Source: CAD feature listing. Evaluate the final solid. Frame: model axes, mm. Face numbers are marked on the shaded views. A direction names the side the tool comes from. Coordinates: 2 decimals unless noted, no trailing zeros. Order: outer loops, then holes, each group sorted by start corner. A loop starts at its lowest first (then second) coordinate and runs counter-clockwise, first axis right, second up. Notation, with made-up numbers: (56, 87) - (81, 87) arc R33 ccw to (81, 123) - close; hole circle Ø7 at (60.25, 84). An arc over 180 degrees is marked (long way). One line per question, with ' | ' between items. Start each with the question number.
(1) Line query: line 1 along Y through (x, z) = (0, 0.15); line 2 along Y through (x, z) = (17.5, 1.05); line 3 along X through (y, z) = (14, -1.7). Output: solid intervals per line, ascending.
(2) Contact query for flat-ended pins moving along their axis: P1, Ø2.5, axis at x = -24.27, y = -14.61, coming from the +Z side; P2, Ø2, axis at y = 7, z = -0.5, coming from the -X side; P3, Ø0.5, axis at x = 10.5, z = -0.5, coming from the -Y side; P4, Ø1.5, axis at x = -12, z = -0.5, coming from the +Y side. Output: stop coordinate, or through.
(3) Section B-B (y = -2.5). Count the separate pieces of the cut face and the enclosed holes in it, then the cut area to 3 significant figures.
(4) Access query for the marked faces 4, 5 and 6. Directions: +Z, -Z, +X, -X, +Y, -Y. A direction counts if a zero-diameter tool reaches every point of the face in a straight line with its end or side. Return the directions, or none.
(5) Draft query along X for the marked faces 1, 2 and 3. Return one class per face: +X half, -X half, draft (parallel to the pull), parting line (faces both ways), or undercut.
(6) Section A-A (x = 0). Return the cut outline in (y, z).
from build123d import *

# Parameters (mm, degrees)
SKETCH_1_R             = 7
SKETCH_1_R_2           = 1.55
EXTRUDE_1_DEPTH        = 2
FILLET_1_R             = 1
CUT_EXTRUDE_START      = -5
CUT_EXTRUDE_1_DEPTH    = 6
FILLET_2_R             = 1
FILLET_2_OF_MIRROR_1_R = 1
SKETCH_3_R             = 1.55
EXTRUDE_2_DEPTH        = 4
FILLET_3_R             = 1
CUT_EXTRUDE_2_DEPTH    = 5
FILLET_4_R             = 1
CUT_EXTRUDE_3_DEPTH    = 5
EXTRUDE_3_DEPTH        = 4
SKETCH_8_R             = 0.75
CUT_EXTRUDE_4_DEPTH    = 5
FILLET_5_R             = 1.5


with BuildPart() as part:
    # 草图1 → 凸台-拉伸1 (new body, symmetric)
    with BuildSketch(Plane.XY):
        with BuildLine():
            Line((-17.5, 11), (-10, 11))
            Line((-10, 11), (-8.321800738, 9))
            Line((-8.321800738, 9), (8.321800738, 9))
            Line((8.321800738, 9), (10, 11))
            Line((10, 11), (17.5, 11))
            ThreePointArc((17.5, 11), (17.577641076, 10.999138732), (17.655243941, 10.99655535))
            Line((17.655243941, 10.99655535), (37, 10.137665421))
            Line((37, 10.137665421), (28.942548731, -12))
            Line((28.942548731, -12), (17.199216279, -10.987051642))
            ThreePointArc((17.199216279, -10.987051642), (15.184578245, -10.124656567), (14.077678472, -8.233290774))
            Line((14.077678472, -8.233290774), (2.304628146, -10.75586766))
            ThreePointArc((2.304628146, -10.75586766), (0, -11), (-2.304628146, -10.75586766))
            Line((-2.304628146, -10.75586766), (-14.077678472, -8.233290774))
            ThreePointArc((-14.077678472, -8.233290774), (-15.184578245, -10.124656567), (-17.199216279, -10.987051642))
            Line((-17.199216279, -10.987051642), (-28.942548731, -12))
            Line((-28.942548731, -12), (-37, 10.137665421))
            Line((-37, 10.137665421), (-17.655243941, 10.99655535))
            ThreePointArc((-17.655243941, 10.99655535), (-17.577641076, 10.999138732), (-17.5, 11))
        make_face()
        Circle(SKETCH_1_R, mode=Mode.SUBTRACT)
        with Locations((17.5, 7.5)):
            Circle(SKETCH_1_R_2, mode=Mode.SUBTRACT)
        with Locations((17.5, -7.5)):
            Circle(SKETCH_1_R_2, mode=Mode.SUBTRACT)
        with Locations((-17.5, -7.5)):
            Circle(SKETCH_1_R_2, mode=Mode.SUBTRACT)
        with Locations((-17.5, 7.5)):
            Circle(SKETCH_1_R_2, mode=Mode.SUBTRACT)
    extrude(amount=EXTRUDE_1_DEPTH, both=True)

    # 圆角1
    fillet_1_edges = [part.edges().sort_by_distance(p)[0] for p in [
        (14.077678472, -8.233290774, 0),
        (-14.077678472, -8.233290774, 0),
    ]]
    fillet(fillet_1_edges, radius=FILLET_1_R)

    # 草图2 → 切除-拉伸1 (cut)
    with BuildSketch(Plane.XY.offset(2).offset(CUT_EXTRUDE_START)):
        Polygon((-20.5, 7.867295251), (-32.782632739, 7.321957304), (-27.222903771, -7.953272497), align=None)
        with BuildLine():
            Line((-19.251811465, 4.412338006), (-24.573190843, -8.11011447))
            Line((-24.573190843, -8.11011447), (-21.036866665, -7.805080632))
            ThreePointArc((-21.036866665, -7.805080632), (-20.623106229, -5.812188553), (-19.182687898, -4.374130291))
            Line((-19.182687898, -4.374130291), (-15.331076504, 4.689613751))
            ThreePointArc((-15.331076504, 4.689613751), (-17.24956823, 3.958844267), (-19.251811465, 4.412338006))
        make_face()
    cut_extrude_1 = extrude(amount=CUT_EXTRUDE_1_DEPTH, mode=Mode.SUBTRACT)

    # 圆角2
    fillet_2_edges = [part.edges().sort_by_distance(p)[0] for p in [
        (-20.5, 7.867295251, 0),
        (-27.222903771, -7.953272497, 0),
        (-32.782632739, 7.321957304, 0),
        (-19.251811465, 4.412338006, 0),
        (-15.331076504, 4.689613751, 0),
        (-19.182687898, -4.374130291, 0),
        (-21.036866665, -7.805080632, 0),
        (-24.573190843, -8.11011447, 0),
    ]]
    fillet(fillet_2_edges, radius=FILLET_2_R)

    # 镜向1: 切除-拉伸1 across plane
    add(cut_extrude_1.mirror(Plane(origin=(0, 0, 0), x_dir=(0, 0, 1), z_dir=(1, 0, 0))), mode=Mode.SUBTRACT)

    # 圆角2 of 镜向1
    fillet_2_of_mirror_1_edges = [part.edges().sort_by_distance(p)[0] for p in [
        (20.5, 7.867295251, 0),
        (27.222903771, -7.953272497, 0),
        (32.782632739, 7.321957304, 0),
        (19.251811465, 4.412338006, 0),
        (15.331076504, 4.689613751, 0),
        (19.182687898, -4.374130291, 0),
        (21.036866665, -7.805080632, 0),
        (24.573190843, -8.11011447, 0),
    ]]
    fillet(fillet_2_of_mirror_1_edges, radius=FILLET_2_OF_MIRROR_1_R)

    # 草图3 → 凸台-拉伸2 (add)
    with BuildSketch(Plane.XY.offset(2)):
        with BuildLine():
            Line((-37.69913918, 12.058534531), (-37, 10.137665421))
            Line((-37, 10.137665421), (-32.4761474, 10.338520445))
            ThreePointArc((-32.4761474, 10.338520445), (-33.315445081, 16.579981486), (-37.69913918, 12.058534531))
        make_face()
        with Locations((-34.410215007, 13.255605032)):
            Circle(SKETCH_3_R, mode=Mode.SUBTRACT)
        with BuildLine():
            Line((-27.557621455, -15.805056417), (-28.942548731, -12))
            Line((-28.942548731, -12), (-22.730405687, -11.464157204))
            ThreePointArc((-22.730405687, -11.464157204), (-21.928391725, -17.210478932), (-27.557621455, -15.805056417))
        make_face()
        with Locations((-24.268697282, -14.607985915)):
            Circle(SKETCH_3_R, mode=Mode.SUBTRACT)
    extrude_2 = extrude(amount=-EXTRUDE_2_DEPTH)

    # 镜向2: 凸台-拉伸2 across plane
    add(extrude_2.mirror(Plane(origin=(0, 0, 0), x_dir=(0, 0, 1), z_dir=(1, 0, 0))))

    # 圆角3
    fillet_3_edges = [part.edges().sort_by_distance(p)[0] for p in [
        (-22.730405687, -11.464157204, 0),
        (-32.4761474, 10.338520445, 0),
        (22.730405687, -11.464157204, 0),
        (32.4761474, 10.338520445, 0),
    ]]
    fillet(fillet_3_edges, radius=FILLET_3_R)

    # 草图4 → 切除-拉伸2 (cut, through all)
    with BuildSketch(Plane.XY.offset(2)):
        with BuildLine():
            Line((-16.384851826, -4.1824038), (-12.057869255, 6))
            Line((-12.057869255, 6), (-8, 6))
            ThreePointArc((-8, 6), (-9.993390733, -0.363512948), (-7.542930102, -6.565379309))
            Line((-7.542930102, -6.565379309), (-15.108699944, -4.944284045))
            ThreePointArc((-15.108699944, -4.944284045), (-15.705867849, -4.49482283), (-16.384851826, -4.1824038))
        make_face()
    cut_extrude_2 = extrude(amount=-CUT_EXTRUDE_2_DEPTH, mode=Mode.SUBTRACT)

    # 镜向3: 切除-拉伸2 across plane
    add(cut_extrude_2.mirror(Plane(origin=(0, 0, 0), x_dir=(0, 0, 1), z_dir=(1, 0, 0))), mode=Mode.SUBTRACT)

    # 圆角4
    fillet_4_edges = [part.edges().sort_by_distance(p)[0] for p in [
        (-12.057869255, 6, 0),
        (-8, 6, 0),
        (-7.542930102, -6.565379309, 0),
        (-15.108699944, -4.944284045, 0),
        (-16.384851826, -4.1824038, 0),
        (8, 6, 0),
        (12.057869255, 6, 0),
        (16.384851826, -4.1824038, 0),
        (15.108699944, -4.944284045, 0),
        (7.542930102, -6.565379309, 0),
    ]]
    fillet(fillet_4_edges, radius=FILLET_4_R)

    # 草图5 → 切除-拉伸3 (cut, through all)
    with BuildSketch(Plane.XY.offset(2)):
        Polygon((30.884976598, -6.370842854), (33.798023723, -7.431105298), (37.25242717, 2.059790172), (34.339380046, 3.120052616), align=None)
    cut_extrude_3 = extrude(amount=-CUT_EXTRUDE_3_DEPTH, mode=Mode.SUBTRACT)

    # 草图7 → 凸台-拉伸3 (add)
    with BuildSketch(Plane.XY.offset(2)):
        Polygon((35.271298659, 5.388097522), (40.439608074, 3.506986734), (35.309305924, -10.588402578), (30.140996509, -8.707291789), (30.97894586, -6.405044868), (33.798023723, -7.431105298), (37.25242717, 2.059790172), (34.433349308, 3.085850601), align=None)
    extrude_3 = extrude(amount=-EXTRUDE_3_DEPTH)

    # 镜向4: 切除-拉伸3, 凸台-拉伸3 across plane
    add(cut_extrude_3.mirror(Plane(origin=(0, 0, 0), x_dir=(0, 0, 1), z_dir=(1, 0, 0))), mode=Mode.SUBTRACT)
    add(extrude_3.mirror(Plane(origin=(0, 0, 0), x_dir=(0, 0, 1), z_dir=(1, 0, 0))))

    # 草图8 → 切除-拉伸4 (cut, through all)
    with BuildSketch(Plane(origin=(0, 0, -2), x_dir=(-1, 0, 0), z_dir=(0, 0, -1))):
        with Locations((-36.995912063, 1.355020706)):
            Circle(SKETCH_8_R)
        with Locations((-34.082864939, 2.41528315)):
            Circle(SKETCH_8_R)
        with Locations((-34.05453883, -6.726335833)):
            Circle(SKETCH_8_R)
        with Locations((-31.141491706, -5.666073389)):
            Circle(SKETCH_8_R)
        with Locations((-35.527813767, 6.092866988)):
            Circle(SKETCH_8_R)
        with Locations((-29.884481402, -9.412061255)):
            Circle(SKETCH_8_R)
    cut_extrude_4 = extrude(amount=-CUT_EXTRUDE_4_DEPTH, mode=Mode.SUBTRACT)

    # 镜向5: 切除-拉伸4 across plane
    add(cut_extrude_4.mirror(Plane(origin=(0, 0, 0), x_dir=(0, 0, 1), z_dir=(1, 0, 0))), mode=Mode.SUBTRACT)

    # 圆角5
    fillet_5_edges = [part.edges().sort_by_distance(p)[0] for p in [
        (40.439608074, 3.506986734, 0),
        (35.309305924, -10.588402578, 0),
        (-40.439608074, 3.506986734, 0),
        (-35.309305924, -10.588402578, 0),
    ]]
    fillet(fillet_5_edges, radius=FILLET_5_R)


solid = part.part
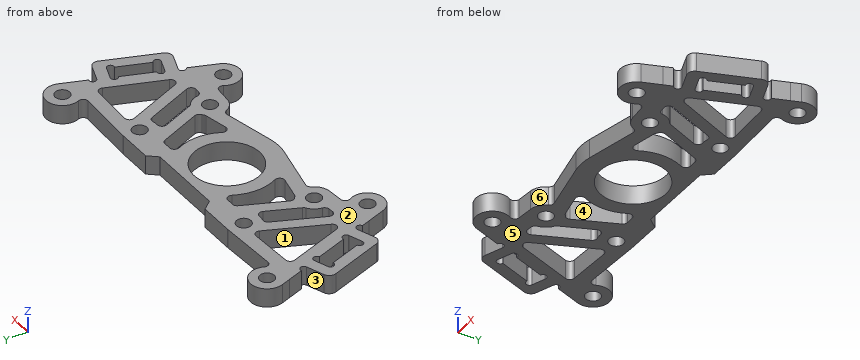
Response values:
1) line 1: y = -11 to -7, 7 to 9 | line 2: y = -11.01 to -9.05, -5.95 to -0.41, 3.95 to 5.95, 9.05 to 11 | line 3: x = -37.83 to -35.77, -33.05 to -30.99, 30.99 to 33.05, 35.77 to 37.83
2) P1: passes through | P2: stops at x = -36.22 | P3: stops at y = -9.05 | P4: stops at y = 11
3) separate pieces: 10 | enclosed holes: 0 | area: 115 mm²
4) face 4: +Z, -Z | face 5: -Z, +X, -X, +Y, -Y | face 6: +Z, -Z, -Y
5) face 1: undercut | face 2: draft | face 3: -X half
6) outline: (-11, -2) - (-7, -2) - (-7, 2) - (-11, 2) - close; (7, -2) - (9, -2) - (9, 2) - (7, 2) - close
